```python
from build123d import *

# Parameters (mm, degrees)
SKETCH_1_W              = 200
SKETCH_1_H              = 213
EXTRUDE_1_DEPTH         = 4
EXTRUDE_2_DEPTH         = 54
CUT_EXTRUDE_2_DEPTH     = 298.880848663
CUT_EXTRUDE_3_DEPTH     = 42
SKETCH_7_R              = 1.8
SKETCH_7_R_2            = 11.5
CUT_EXTRUDE_4_DEPTH     = 282.53330176
MIRROR_START            = 176
MIRROR_1_OUTLINE_R      = 1.8
MIRROR_1_OUTLINE_R_2    = 11.5
MIRROR_1_DEPTH          = 3.5
CUT_EXTRUDE_START       = -21
CUT_EXTRUDE_5_OUTLINE_W = 27
CUT_EXTRUDE_5_OUTLINE_H = 20
CUT_EXTRUDE_5_DEPTH     = 21
CUT_EXTRUDE_START_2     = -6
CUT_EXTRUDE_6_OUTLINE_W = 27
CUT_EXTRUDE_6_OUTLINE_H = 28
CUT_EXTRUDE_6_DEPTH     = 6
CUT_EXTRUDE_START_3     = -54
CUT_EXTRUDE_7_DEPTH     = 54
SKETCH_12_R             = 2
EXTRUDE_3_DEPTH         = 10


# Read off the part's stored shape, not the designer's step: 镜向1, 切除-拉伸5, 切除-拉伸6
with BuildPart() as part:
    # 草图1 → 凸台-拉伸1 (new body)
    with BuildSketch(Plane(origin=(0, 0, 0), x_dir=(1, 0, 0), z_dir=(0, 1, 0))):
        with Locations((100, 106.5)):
            Rectangle(SKETCH_1_W, SKETCH_1_H)
    extrude(amount=EXTRUDE_1_DEPTH)

    # 草图1<4> → 凸台-拉伸2 (add)
    with BuildSketch(Plane(origin=(0, 0, 0), x_dir=(1, 0, 0), z_dir=(0, 1, 0))):
        with BuildLine():
            Line((0, 213), (0, 0))
            ThreePointArc((0, 0), (21.966991411, 53.033008589), (75, 75))
            Line((75, 75), (75, 213))
            Line((75, 213), (0, 213))
        make_face()
        with BuildLine():
            Line((125, 213), (125, 75))
            ThreePointArc((125, 75), (178.033008589, 53.033008589), (200, 0))
            Line((200, 0), (200, 213))
            Line((200, 213), (125, 213))
        make_face()
    extrude(amount=-EXTRUDE_2_DEPTH)

    # 草图3 → 切除-拉伸2 (cut, through all)
    with BuildSketch(Plane.XZ.offset(54)):
        Polygon((20.5, -186), (20.5, -165), (20.5, -144), (20.5, -115), (0, -115), (0, -213), (20.5, -213), align=None)
        Polygon((179.5, -115), (200, -115), (200, -213), (179.5, -213), (179.5, -165), align=None)
    extrude(amount=-CUT_EXTRUDE_2_DEPTH, mode=Mode.SUBTRACT)

    # 草图5 → 切除-拉伸3 (cut)
    with BuildSketch(Plane.XZ.offset(54)):
        Polygon((176, -164), (176, -144), (125, -144), (125, -186), (176, -186), align=None)
        Polygon((24, -164), (24, -144), (75, -144), (75, -186), (24, -186), align=None)
    extrude(amount=-CUT_EXTRUDE_3_DEPTH, mode=Mode.SUBTRACT)

    # 草图7 → 切除-拉伸4 (cut, through all)
    with BuildSketch(Plane(origin=(24, 0, 0), x_dir=(0, 0, -1), z_dir=(1, 0, 0))):
        with Locations((180.5, -17.5)):
            Circle(SKETCH_7_R)
        with Locations((149.5, -17.5)):
            Circle(SKETCH_7_R)
        with Locations((165, -33)):
            Circle(SKETCH_7_R_2)
        with Locations((180.5, -48.5)):
            Circle(SKETCH_7_R)
        with Locations((149.5, -48.5)):
            Circle(SKETCH_7_R)
    extrude(amount=-CUT_EXTRUDE_4_DEPTH, mode=Mode.SUBTRACT)

    # 镜向1 outline → 镜向1 (cut)
    with BuildSketch(Plane.YZ.offset(MIRROR_START)):
        with Locations((-17.5, -180.5)):
            Circle(MIRROR_1_OUTLINE_R)
        with Locations((-17.5, -149.5)):
            Circle(MIRROR_1_OUTLINE_R)
        with Locations((-33, -165)):
            Circle(MIRROR_1_OUTLINE_R_2)
        with Locations((-48.5, -180.5)):
            Circle(MIRROR_1_OUTLINE_R)
        with Locations((-48.5, -149.5)):
            Circle(MIRROR_1_OUTLINE_R)
    extrude(amount=MIRROR_1_DEPTH, mode=Mode.SUBTRACT)

    # 切除-拉伸5 outline → 切除-拉伸5 (cut)
    with BuildSketch(Plane(origin=(75, 0, 0), x_dir=(0, 0, -1), z_dir=(1, 0, 0)).offset(CUT_EXTRUDE_START)):
        with Locations((199.5, -33)):
            Rectangle(CUT_EXTRUDE_5_OUTLINE_W, CUT_EXTRUDE_5_OUTLINE_H)
    extrude(amount=CUT_EXTRUDE_5_DEPTH, mode=Mode.SUBTRACT)

    # 切除-拉伸6 outline → 切除-拉伸6 (cut)
    with BuildSketch(Plane.ZY.offset(-125).offset(CUT_EXTRUDE_START_2)):
        with Locations((-199.5, -33)):
            Rectangle(CUT_EXTRUDE_6_OUTLINE_W, CUT_EXTRUDE_6_OUTLINE_H)
    extrude(amount=CUT_EXTRUDE_6_DEPTH, mode=Mode.SUBTRACT)

    # 草图11 → 切除-拉伸7 (cut)
    with BuildSketch(Plane.XZ.offset(54).offset(CUT_EXTRUDE_START_3)):
        with BuildLine():
            Line((29.658534166, -69.684244774), (10.975621098, -39.0625))
            ThreePointArc((10.975621098, -39.0625), (38.289562111, -65.401404801), (75, -75))
            Line((75, -75), (75, -144))
            ThreePointArc((75, -144), (37.483837038, -124.777752739), (31.171635941, -83.099060455))
            ThreePointArc((31.171635941, -83.099060455), (31.899182276, -76.224256342), (29.658534166, -69.684244774))
        make_face()
        with BuildLine():
            Line((125, -144), (125, -75))
            ThreePointArc((125, -75), (161.710437889, -65.401404801), (189.024378902, -39.0625))
            Line((189.024378902, -39.0625), (170.341465834, -69.684244774))
            ThreePointArc((170.341465834, -69.684244774), (168.100817724, -76.224256342), (168.828364059, -83.099060455))
            ThreePointArc((168.828364059, -83.099060455), (162.516162962, -124.777752739), (125, -144))
        make_face()
    extrude(amount=CUT_EXTRUDE_7_DEPTH, mode=Mode.SUBTRACT)

    # 草图12 → 凸台-拉伸3 (add)
    # profile 1 of 2: a face of its own
    with BuildSketch(Plane.XZ.offset(54)):
        with BuildLine():
            Line((18.008349917, -58.289006678), (26.711199556, -66.131863821))
            ThreePointArc((26.711199556, -66.131863821), (32, -78.017578107), (26.711199556, -89.903292393))
            Line((26.711199556, -89.903292393), (18.008349917, -97.746149535))
            ThreePointArc((18.008349917, -97.746149535), (16, -98.517578107), (13.991650083, -97.746149535))
            Line((13.991650083, -97.746149535), (5.288800444, -89.903292393))
            ThreePointArc((5.288800444, -89.903292393), (0, -78.017578107), (5.288800444, -66.131863821))
            Line((5.288800444, -66.131863821), (13.991650083, -58.289006678))
            ThreePointArc((13.991650083, -58.289006678), (16, -57.517578107), (18.008349917, -58.289006678))
        make_face()
        with Locations(Location((16, -60.517578107, 0), (0, 0, 270))):
            Circle(SKETCH_12_R, mode=Mode.SUBTRACT)
        with Locations(Location((16, -95.517578107, 0), (0, 0, 90))):
            Circle(SKETCH_12_R, mode=Mode.SUBTRACT)
    # profile 2 of 2: a face of its own
    with BuildSketch(Plane.XZ.offset(54)):
        with BuildLine():
            Line((186.008349917, -97.746149535), (194.711199556, -89.903292393))
            ThreePointArc((194.711199556, -89.903292393), (200, -78.017578107), (194.711199556, -66.131863821))
            Line((194.711199556, -66.131863821), (186.008349917, -58.289006678))
            ThreePointArc((186.008349917, -58.289006678), (184, -57.517578107), (181.991650083, -58.289006678))
            Line((181.991650083, -58.289006678), (173.288800444, -66.131863821))
            ThreePointArc((173.288800444, -66.131863821), (168, -78.017578107), (173.288800444, -89.903292393))
            Line((173.288800444, -89.903292393), (181.991650083, -97.746149535))
            ThreePointArc((181.991650083, -97.746149535), (184, -98.517578107), (186.008349917, -97.746149535))
        make_face()
        with Locations(Location((184, -95.517578107, 0), (0, 0, 270))):
            Circle(SKETCH_12_R, mode=Mode.SUBTRACT)
        with Locations(Location((184, -60.517578107, 0), (0, 0, 90))):
            Circle(SKETCH_12_R, mode=Mode.SUBTRACT)
    extrude(amount=EXTRUDE_3_DEPTH)


solid = part.part
```
Geometry: final body of the model. Coordinates: model frame, mm. A direction names the side the tool comes from. Coordinates: 2 decimals unless noted, no trailing zeros. Order: outer loops, then holes, each group sorted by start corner. A loop starts at its lowest first (then second) coordinate and runs counter-clockwise, first axis right, second up. Notation, with made-up numbers: (-14.5, 58) -> (6.5, 58) arc R19 ccw to (6.5, 76) -> close; hole circle Ø10 at (31, 39). An arc over 180 degrees is marked (long way). Write each question's results on one line, items separated by ' | '. Start each with the question number.
1) Cut plane C-C, the plane z = -123. Output: boundary loops of the cut face in (x, y).
2) Cut plane D-D, the plane z = -52. Output: boundary loops of the cut face in (x, y), and give its area (3 significant figures).
3) First-contact query: pin 1 (3 mm diameter, centred on y = -17.5, z = -149.5, fed in from +X); pin 2 (1 mm diameter, centred on y = -9.5, z = -186.5, fed in from -X); pin 3 (2 mm diameter, centred on x = 61.5, z = -52.5, fed in from -Y); pin 4 (6 mm diameter, centred on y = -48.5, z = -180.5, fed in from +X). Flat tips, straight axial feed; report the tip coordinate or a pass-through.
4) Set-up query: faces 1 (the flat face through (64, -23, -199)), 2 (the flat face through (176, -24, -156)), 3 (the flat face through (75, -48, -199)), 4 (the flat face through (190.3, -58.93, -93.88)), 5 (the flat face through (9.7, -58.93, -93.88)). Return all of +Z, -Z, +X, -X, +Y, -Y with unobstructed straight access to the full face (end or side cutting, diameter ignored); none if empty.
5) Cut plane A-A, the plane z = -165. Output: boundary loops of the cut face in (x, y), and give its area (3 significant figures).
6) Cut plane B-B, the plane x = 72.5. Output: boundary loops of the cut face in (y, z), and give its area (3 significant figures).
7) Mould query, pull axis Z, two halves, no side actions, for faces 6 (the flat face through (128, -47, -200)), 7 (the cylindrical face through (0, -59, -78)), 8 (the flat face through (151, -33, -144)), 9 (the flat face through (190, -25, -115)). Classes: released by +Z, released by -Z, zero draft, split by the parting line, or undercut.
8) Material intervals for line 1 along Z through (x, y) = (184, -56.25); line 2 along Y through (x, z) = (64.5, -189.5); line 3 along X through (y, z) = (-37, -200.5), sorted ascending.
Checks:
1) outline: (20.5, -54) -> (36.27, -54) -> (36.27, 0) -> (163.73, 0) -> (163.73, -54) -> (179.5, -54) -> (179.5, 4) -> (20.5, 4) -> close
2) outline: (0, -54) -> (18.87, -54) -> (18.87, 0) -> (181.13, 0) -> (181.13, -54) -> (200, -54) -> (200, 4) -> (0, 4) -> close | area: 2,840 mm^2
3) pin 1: through | pin 2: x = 20.5 | pin 3: y = 0 | pin 4: x = 179.5
4) face 1: -Z | face 2: -Y | face 3: +Z, -Z, -Y | face 4: -Z, +X, -Y | face 5: -Z, -X, -Y
5) outline: (20.5, -54) -> (24, -54) -> (24, -44.5) -> (20.5, -44.5) -> close; (20.5, -21.5) -> (24, -21.5) -> (24, -12) -> (75, -12) -> (75, 0) -> (125, 0) -> (125, -12) -> (176, -12) -> (176, -21.5) -> (179.5, -21.5) -> (179.5, 4) -> (20.5, 4) -> close; (176, -54) -> (179.5, -54) -> (179.5, -44.5) -> (176, -44.5) -> close | area: 2,080 mm^2
6) outline: (-54, -213) -> (-43, -213) -> (-43, -186) -> (-54, -186) -> close; (-54, -144) -> (-12, -144) -> (-12, -186) -> (-23, -186) -> (-23, -213) -> (4, -213) -> (4, 0) -> (0, 0) -> (0, -143.93) -> (-54, -143.93) -> close | area: 2,280 mm^2
7) face 6: zero draft | face 7: split by the parting line | face 8: undercut | face 9: released by -Z
8) line 1: -98.52 to -97.52, -93.52 to -62.52, -58.52 to -57.52 | line 2: -54 to -43, -23 to 4 | line 3: 20.5 to 54, 131 to 179.5
